Geometry: final body of the model. Coordinates: model frame, mm. Face numbers are marked on the shaded views. Round coordinates to 2 decimals unless told otherwise and drop trailing zeros. Loops run counter-clockwise (first coordinate to the right, second up) from the corner with the lowest first, then second, coordinate; pieces in that order, holes last. Notation, with made-up numbers: M 21,-5.5 L 75,-5.5 A14 cw 75,12.5 Z; hole C -34.75,-1 d9. An arc over 180 degrees is marked long. Answer as a JSON object with one key per item and string values.
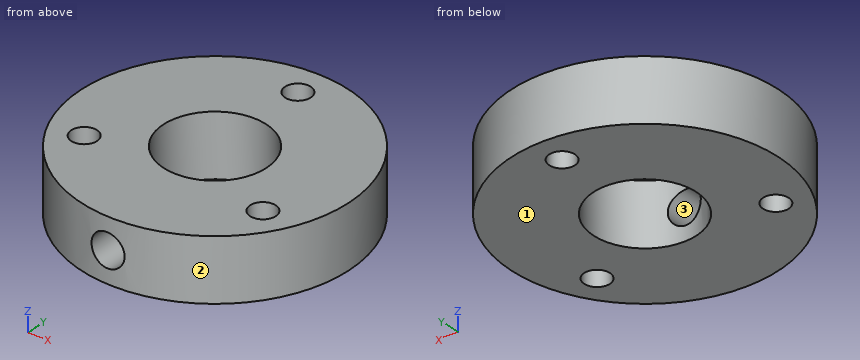
```python
from build123d import *

# Parameters (mm, degrees)
MODEL_R             = 6.5
EXTRUDE_338_DEPTH   = 1.5
SKETCH_3_R          = 2.5
CUT_EXTRUDE_1_DEPTH = 10.669539803
HOLE_WIZARD_M1_6_D  = 1.25
SKETCH_8_W          = 0.8
SKETCH_8_H          = 6.5


with BuildPart() as part:
    # Model → Extrude 338 (new, symmetric)
    with BuildSketch(Plane.XY):
        Circle(MODEL_R)
    extrude(amount=EXTRUDE_338_DEPTH, both=True)

    # Эскиз3 → Вырез-Вытянуть1 (cut, through all)
    with BuildSketch(Plane.XY.offset(1.5)):
        Circle(SKETCH_3_R)
    extrude(amount=-CUT_EXTRUDE_1_DEPTH, mode=Mode.SUBTRACT)

    # Крепление шестерни M1.6 (through all)
    with Locations(Plane.XY.offset(1.5)):
        with Locations((0, 5), (4.330127019, -2.5), (-4.330127019, -2.5)):
            Hole(HOLE_WIZARD_M1_6_D / 2)

    # Эскиз8 → Крепление на вал M2 (revolve, cut)
    with BuildSketch(Plane(origin=(0, 0, 0), x_dir=(0, 0, 1), z_dir=(1, 0, 0))):
        with Locations((0.4, 3.25)):
            Rectangle(SKETCH_8_W, SKETCH_8_H)
    revolve(axis=Axis((0, 6.35, 0), (0, -1, 0)), mode=Mode.SUBTRACT)


solid = part.part
```
1) Cut plane A-A on x = 0. Return the cut outline in (y, z) (3 decimals).
Geometry results:
{"outline": "M -6.5,-1.5 L -2.5,-1.5 L -2.5,-0.8 L -6.5,-0.8 Z; M -6.5,0.8 L -2.5,0.8 L -2.5,1.5 L -6.5,1.5 Z; M 2.5,-1.5 L 4.375,-1.5 L 4.375,1.5 L 2.5,1.5 Z; M 5.625,-1.5 L 6.5,-1.5 L 6.5,1.5 L 5.625,1.5 Z"}
2) Line query: probe 1 along Z at (x, y) = (0, -3.7); probe 2 along Y at (x, z) = (0, -1.15) (3 decimals); probe 3 along X at (y, z) = (-6, -0.95). Output: solid intervals per line, ascending.
Geometry results:
{"probe 1": "-1.5 to -0.8, 0.8 to 1.5", "probe 2": "-6.5 to -2.5, 2.5 to 4.375, 5.625 to 6.5", "probe 3": "-2.5 to 2.5"}
3) Cut plane B-B on z = 0. Return the cut outline in (x, y) (3 decimals), and give its area (3 significant figures).
Geometry results:
{"outline": "M -0.8,-6.451 L -0.8,-2.369 A2.5 cw long 0.8,-2.369 L 0.8,-6.451 A6.5 ccw long Z; hole C -4.33,-2.5 d1.25; hole C 0,5 d1.25; hole C 4.33,-2.5 d1.25", "area": "103 mm2"}
4) Pull-direction query (X, two-part tool) for the marked faces 1, 2 and 3; classes: +X half, -X half, draft (parallel to the pull), parting line (faces both ways), or undercut.
Geometry results:
{"face 1": "draft", "face 2": "parting line", "face 3": "undercut"}
5) Cut plane D-D on z = 1. Return the cut outline in (x, y) (3 decimals), and give its area (3 significant figures).
Geometry results:
{"outline": "C 0,0 d13; hole C -4.33,-2.5 d1.25; hole C 0,0 d5; hole C 0,5 d1.25; hole C 4.33,-2.5 d1.25", "area": "109 mm2"}
6) First-contact query: pin 1 (1.5 mm diameter, centred on x = -1, z = 0.5, fed in from +Y); pin 2 (1.1 mm diameter, centred on x = 4.33, y = -2.5, fed in from -Z). Flat tips, straight axial feed; report the tip coordinate or a pass-through.
Geometry results:
{"pin 1": "y = 6.5", "pin 2": "through"}
7) Cut plane C-C on y = -0.5. Return the cut outline in (x, z).
Geometry results:
{"outline": "M -6.48,-1.5 L -2.45,-1.5 L -2.45,1.5 L -6.48,1.5 Z; M 2.45,-1.5 L 6.48,-1.5 L 6.48,1.5 L 2.45,1.5 Z"}
